Autodesk Inventor part; units mm, degrees
ref_plane "YZ Plane" through (0, 0, 0) normal (1, 0, 0) x (0, 1, 0)
ref_plane "XZ Plane" through (0, 0, 0) normal (0, 1, 0) x (-1, 0, 0)
ref_plane "XY Plane" through (0, 0, 0) normal (0, 0, 1) x (1, 0, 0)
sketch "Sketch1" plane through (0, 0, 0) normal (1, 0, 0) x (0, 1, 0)
  line L0 (-5, 25) -> (5, 25)
  line L1 (5, 25) -> (5, -25)
  line L2 (5, -25) -> (-5, -25)
  line L3 (-5, -25) -> (-5, 25)
  line L4 (-5, 25) -> (5, -25) construction
  line L5 (5, 25) -> (-5, -25) construction
  line L6 (-5, -25) -> (-15, -25)
  line L7 (-15, -25) -> (-15, -15)
  line L8 (-15, -15) -> (-5, -15)
  line L9 (-5, -15) -> (-5, -25)
  line L10 (5, 0) -> (-34.0233, 0) construction
  line L11 (-5, 25) -> (-15, 25)
  line L12 (-15, 25) -> (-15, 15)
  line L13 (-15, 15) -> (-5, 15)
  point P0 (0, 0)
  point P1 (-15, -20)
  dimension "d0" = 50
  dimension "d1" = 10
  dimension "d2" = 10
  dimension "d3" = 20
extrude "Extrusion1" add sketch "Sketch1" along normal mid plane 90
sketch "Sketch2" plane through (45, 5, -25) normal (0, 0, -1) x (-1, 0, 0)
  line L0 (0, 0) -> (90, 0)
  line L1 (0, -20) -> (0, 0)
  line L2 (90, -20) -> (0, -20)
  line L3 (90, 0) -> (90, -20)
  line L4 (15, 0) -> (75, 0)
  line L5 (75, 0) -> (75, 30)
  line L6 (75, 30) -> (15, 30)
  line L7 (15, 30) -> (15, 0)
  point P0 (45, -5)
  point P1 (45, 30)
  dimension "d6" = 50
  dimension "d7" = 60
extrude "Extrusion2" add sketch "Sketch2" against normal blind 10 contours L7 L6 L5 L0
sketch "Sketch3" plane through (-30, 5, -25) normal (-1, 0, 0) x (0, 0, 1)
  line L0 (0, 30) -> (10, 30)
  line L1 (0, 0) -> (50, 0)
  line L2 (10, 30) -> (50, 10)
  line L3 (50, 0) -> (50, -20)
  line L4 (50, 0) -> (50, 10)
  line L5 (40, -20) -> (50, -20)
  line L6 (0, 0) -> (0, 30)
  point P0 (25, -5)
  dimension "d28" = 30
extrude "Extrusion4" add sketch "Sketch3" against normal blind 10
mirror "Mirror1" about plane through (0, 0, 0) normal (1, 0, 0) of "Extrusion4"
sketch "Sketch4" plane through (45, 5, -15) normal (0, 0, 1) x (1, 0, 0)
  circle A0 centre (-45, 20) radius 10
  line L0 (-55, 20) -> (-55, 30)
  line L1 (-15, 30) -> (-75, 30)
  line L2 (-45, 30) -> (-45, 0) construction
  line L3 (-15, 0) -> (-75, 0)
  line L4 (-35, 20) -> (-35, 30)
  point P0 (-45, -5)
  point P1 (-25, 30)
  point P2 (-65, 30)
  point P3 (-25, 0)
  point P4 (-65, 0)
  point P5 (-45, 10)
  point P6 (-35, 20)
  dimension "d16" = 20
  dimension "d17" = 20
extrude "Extrusion3" cut sketch "Sketch4" against normal through all
sketch "Sketch5" plane through (-20, 5, 25) normal (0, 1, 0) x (1, 0, 0)
  line L0 (40, 40) -> (30, 40)
  line L1 (0, 0) -> (40, 0)
  point P0 (20, 20)
  point P1 (50, 40)
  point P2 (20, 0)
  dimension "d20" = 20
hole "Hole1" at (0, 5, 5) direction (0, -1, 0) diameter 20 end through all
properties part number "s14-12"
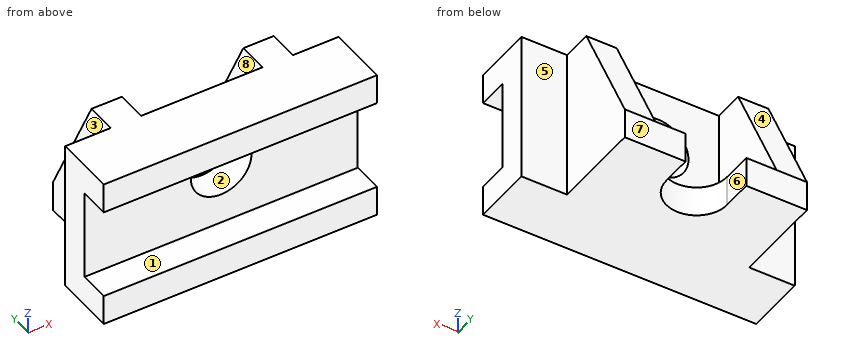
Input: part model. Units: mm. Frame: model coordinates. Face numbers are marked on the shaded views. A direction names the side the tool comes from. Round coordinates to 2 decimals unless told otherwise and drop trailing zeros. Loops run counter-clockwise (first coordinate to the right, second up) from the corner with the lowest first, then second, coordinate; pieces in that order, holes last. Notation, with made-up numbers: (70, -7) -> (124, -7) arc R12 cw to (124, 3) -> close; hole circle Ø3 at (-32, 48.25). An arc over 180 degrees is marked (long way). Answer as a JSON object with one key per item and string values. Group by question number.
1) Section query B-B on z = 5. Output: boundary loops of the cut face in (x, y), plus the area to 3 significant figures.
2) Section query D-D on x = -14. Output: boundary loops of the cut face in (y, z).
3) Ray query, L1, parallel to Z at x = 32.5, y = -11; L2, parallel to X at y = -2.5, z = 5; L3, parallel to Z at x = 0, y = -3. Return the intervals inside material, ascending.
4) Section query A-A on y = -6. Output: boundary loops of the cut face in (x, z).
5) Pin query (flat end, axial travel): pin 1 (7.5 mm diameter, centred on x = -34, z = -7.5, fed in from +Y); pin 2 (8 mm diameter, centred on y = 30, z = -20, fed in from -X); pin 3 (1 mm diameter, centred on x = 26.5, z = -3, fed in from -Y). Return the tip coordinate at first contact, or that it passes through.
6) Draft query along Z for the marked faces 1, 2, 3 and 4. Return one class per face: +Z half, -Z half, draft (parallel to the pull), parting line (faces both ways), or undercut.
7) Section query C-C on x = 1. Output: boundary loops of the cut face in (y, z), plus the area to 3 significant figures.
8) Reachability of the marked faces 5, 6, 7 and 8 from +Z, -Z, +X, -X, +Y, -Y: full face, straight path, thin tool, end or side. Return the list, or none.
Reply:
{
 "1": {"outline": "(-45, -5) -> (-10, -5) -> (-10, 5) -> (-20, 5) -> (-20, 25) -> (-30, 25) -> (-30, 5) -> (-45, 5) -> close; (10, -5) -> (45, -5) -> (45, 5) -> (30, 5) -> (30, 25) -> (20, 25) -> (20, 5) -> (10, 5) -> close", "area": "1,100 mm2"},
 "2": {"outline": "(-15, -25) -> (35, -25) -> (35, -15) -> (5, -15) -> (5, 25) -> (-15, 25) -> (-15, 15) -> (-5, 15) -> (-5, -15) -> (-15, -15) -> close"},
 "3": {"L1": "z = -25 to -15, 15 to 25", "L2": "x = -45 to -10, 10 to 45", "L3": "z = -25 to -5, 15 to 25"},
 "4": {"outline": "(-45, -25) -> (45, -25) -> (45, -15) -> (-45, -15) -> close; (-45, 15) -> (45, 15) -> (45, 25) -> (-45, 25) -> close"},
 "5": {"pin 1": "stops at y = 5", "pin 2": "stops at x = -30", "pin 3": "stops at y = -5"},
 "6": {"face 1": "undercut", "face 2": "undercut", "face 3": "draft", "face 4": "+Z half"},
 "7": {"outline": "(-15, -25) -> (15.05, -25) -> (15.05, -15) -> (5, -15) -> (5, -4.95) -> (-5, -4.95) -> (-5, -15) -> (-15, -15) -> close; (-15, 15) -> (-5, 15) -> (-5, 14.95) -> (5, 14.95) -> (5, 25) -> (-15, 25) -> close", "area": "602 mm2"},
 "8": {"face 5": "+Z, -Z, +X, +Y", "face 6": "+Z, -Z, +Y", "face 7": "+Z, -Z, +X, -X, +Y", "face 8": "+Z, +Y"}
}
